Could you check a few things on this model? Use its own coordinates, in mm. A direction names the side the tool comes from. Give positions to 0.01 mm unless a question says otherwise; leave off trailing zeros. Write each loop counter-clockwise with the first axis right and the second up, starting at its lowest first coordinate (ties: lowest second). Pieces come first, ordered by that corner, then holes. Notation, with made-up numbers: (30, -28.5) - (66, -28.5) arc R19 cw to (66, -14.5) - close; hole circle Ø8 at (45.5, 60.25). An arc over 180 degrees is marked (long way). Answer in a Markdown table with one row per item.
Autodesk Inventor part; units mm, degrees
ref_plane "Work Plane1" through (0, 0, 47) normal (0, 0, -1) x (-1, 0, 0)
ref_plane "YZ Plane" through (0, 0, 0) normal (1, 0, 0) x (0, 1, 0)
ref_plane "XZ Plane" through (0, 0, 0) normal (0, 1, 0) x (-1, 0, 0)
sketch "Sketch1" plane through (0, 0, 0) normal (0, 0, 1) x (1, 0, 0)
  circle A0 centre (0, 0) radius 4
  dimension "d0" = 8
extrude "Extrusion1" add sketch "Sketch1" along normal blind 94
sketch "Sketch2" plane through (0, 0, 94) normal (0, 0, 1) x (1, 0, 0)
  circle A0 centre (0, 0) radius 1.5
  dimension "d3" = 3
extrude "Extrusion2" cut sketch "Sketch2" against normal blind 20
ref_plane "Work Plane1" through (0, 0, 47) normal (0, 0, -1) x (-1, 0, 0)
mirror "Mirror1" about plane through (0, 0, 47) normal (0, 0, -1) of "Extrusion2"
properties part number "BatteryHolderRod"
1) If I drill on line 1 (Y direction, x = 0, z = 79); line 2 (Z direction, x = 1, y = -0.5); line 3 (X direction, y = 0.25, z = 69), over which ranges is the centre line in solid material (lowest first)?
Check values:
| item | result |
|---|---|
| line 1 | y = -4 to -1.5, 1.5 to 4 |
| line 2 | z = 20 to 74 |
| line 3 | x = -3.99 to 3.99 |
2) Imagine slicing it at B-B (z = 17). List the corners of the cut face in (x, y) for me, then the cut area to 3 significant figures.
Check values:
| item | result |
|---|---|
| outline | circle Ø8 at (0, 0); hole circle Ø3 at (0, 0) |
| area | 43.2 mm2 |
3) Imagine slicing it at A-A (x = 0). List the corners of the cut face in (y, z) for me.
Check values:
| item | result |
|---|---|
| outline | (-4, 0) - (-1.5, 0) - (-1.5, 20) - (1.5, 20) - (1.5, 0) - (4, 0) - (4, 94) - (1.5, 94) - (1.5, 74) - (-1.5, 74) - (-1.5, 94) - (-4, 94) - close |
4) Imagine slicing it at D-D (z = 53). List the corners of the cut face in (x, y) for me, then the cut area to 3 significant figures.
Check values:
| item | result |
|---|---|
| outline | circle Ø8 at (0, 0) |
| area | 50.3 mm2 |
5) On a 3-axis mill with a long thin cutter (end or side, diameter ignored), from which of +Z, -Z, +X, -X, +Y, -Y can I reach the whole of each face in a straight line? I mean faces 1 (the face through (0, 0, 74)), 2 (the face through (0, 0, 20)), 3 (the face through (2, 0, 94)). Say none if no direction works.
Check values:
| item | result |
|---|---|
| face 1 | +Z |
| face 2 | -Z |
| face 3 | +Z, +X, -X, +Y, -Y |
6) We'd pull the mould along Y, two halves only. Please class faces 4 (the face through (-0.867, 3.905, 46.342)), 5 (the face through (-1.5, -0.07, 9.86)), 6 (the face through (2, 0, 0)), 7 (the face through (-1.5, 0.07, 84.14)): +Y half, -Y half, draft (parallel to the pull), parting line (faces both ways), or undercut.
Check values:
| item | result |
|---|---|
| face 4 | parting line |
| face 5 | undercut |
| face 6 | draft |
| face 7 | undercut |
7) Will these pins go through, and if not, where does the flat tip stop? P1, Ø1.5, axis at x = 0.5, y = 0.5, coming from the -Z side; P2, Ø2.5, axis at x = 0, y = 0, coming from the +Z side; P3, Ø3, axis at x = -2.5, z = 23, coming from the -Y side.
Check values:
| item | result |
|---|---|
| P1 | stops at z = 20 |
| P2 | stops at z = 74 |
| P3 | stops at y = -3.87 |
